Part print with two shaded views. Sizes in mm from the minimum x, y, z corner. Round coordinates to 2 decimals unless told otherwise and drop trailing zeros. Write each loop counter-clockwise with the first axis right and the second up, starting at its lowest first coordinate (ties: lowest second). Pieces come first, ordered by that corner, then holes. Notation, with made-up numbers: (84.25, 86) - (88.25, 86) arc R11 cw to (88.25, 101) - close; hole circle Ø1 at (62, 66.5). An arc over 180 degrees is marked (long way). Use one line per item in the form item = value. Start each with the question number.
Item 1: Band-saw the part on B-B, the plane z = 5.5. List the corners of the cut face in (x, y).
Item 2: Band-saw the part on C-C, the plane y = 1. List the corners of the cut face in (x, z), and give its area (3 significant figures).
Item 3: Band-saw the part on A-A, the plane x = 10. List the corners of the cut face in (y, z), and give its area (3 significant figures).
Item 4: Band-saw the part on D-D, the plane z = 13.25. List the corners of the cut face in (x, y), and give its area (3 significant figures).
Item 5: Pin check, flat tip, straight feed: pin 1 (1 mm diameter, centred on y = 4, z = 9, fed in from -X). Stop position of the tip, or through.
Item 6: Pull direction X, two halves, no side cores. Call the marked faces 1, 2, 3 and 4: +X half, -X half, draft (parallel to the pull), parting line (faces both ways), or undercut.
Item 7: Drill centre lines: L1, parallel to X at y = 5.25, z = 7.5; L2, parallel to X at y = 2.25, z = 6.25; L3, parallel to Z at x = 5, y = 2.5. Where is each one in solid material? Low to high.
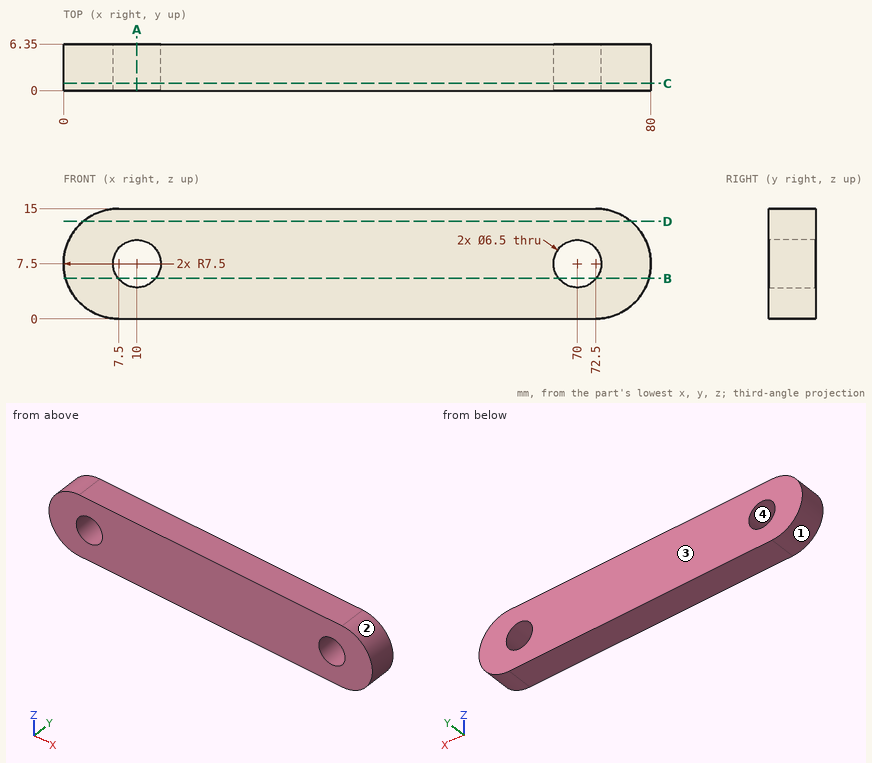
Determined:
q1.outline = (0.27, 0) - (7.44, 0) - (7.44, 6.35) - (0.27, 6.35) - close; (12.56, 0) - (67.44, 0) - (67.44, 6.35) - (12.56, 6.35) - close; (72.56, 0) - (79.73, 0) - (79.73, 6.35) - (72.56, 6.35) - close
q2.outline = (7.5, 0) - (72.5, 0) arc R7.5 ccw to (72.5, 15) - (7.5, 15) arc R7.5 ccw to start; hole circle Ø6.5 at (10, 7.5); hole circle Ø6.5 at (70, 7.5)
q2.area = 1,090 mm²
q3.outline = (0, 0) - (6.35, 0) - (6.35, 4.25) - (0, 4.25) - close; (0, 10.75) - (6.35, 10.75) - (6.35, 15) - (0, 15) - close
q3.area = 54.0 mm²
q4.outline = (2.68, 0) - (77.32, 0) - (77.32, 6.35) - (2.68, 6.35) - close
q4.area = 474 mm²
q5.pin_1 = 0.07
q6.face_1 = -X half
q6.face_2 = +X half
q6.face_3 = draft
q6.face_4 = undercut
q7.L1 = 0 to 6.75, 13.25 to 66.75, 73.25 to 80
q7.L2 = 0.1 to 7, 13 to 67, 73 to 79.9
q7.L3 = 0.43 to 14.57
